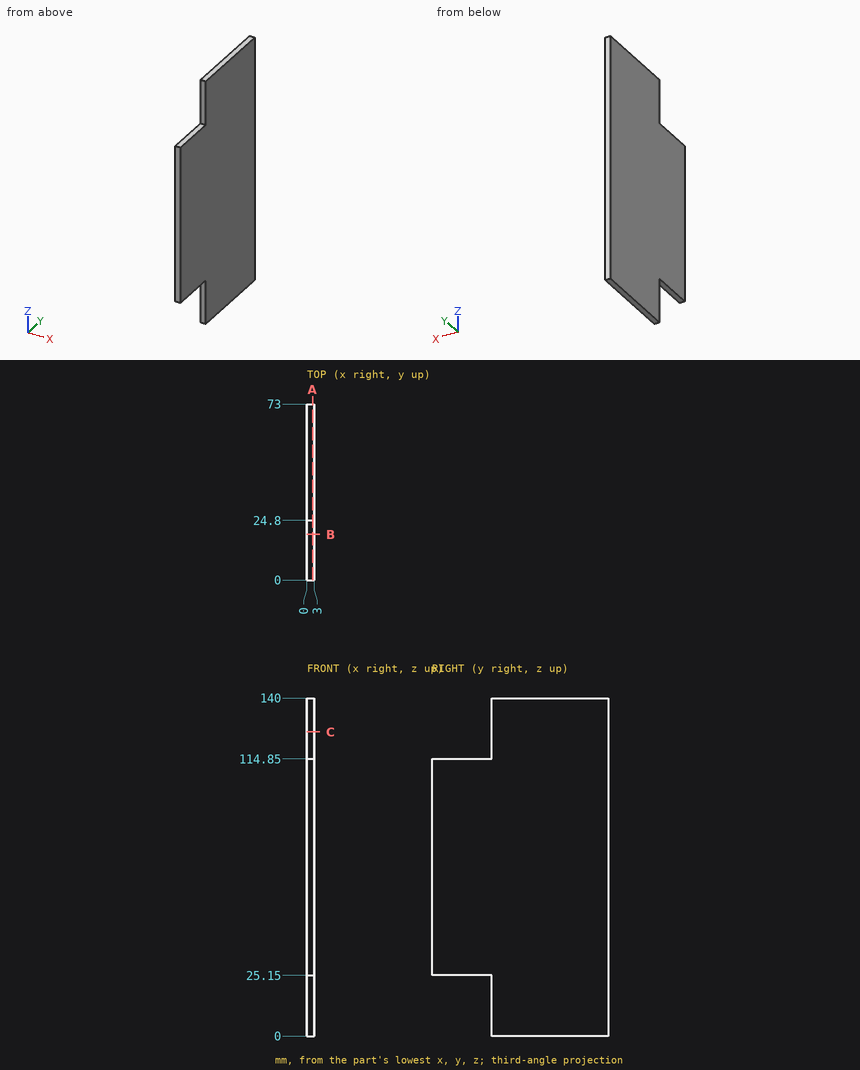
Can you work these out from the drawing? Everything is in mm from the part's minimum corner. Round coordinates to 2 decimals unless told otherwise and drop trailing zeros. Loops run counter-clockwise (first coordinate to the right, second up) from the corner with the lowest first, then second, coordinate; pieces in that order, holes last. Notation, with made-up numbers: (29, 76.5) - (78, 76.5) arc R18 ccw to (78, 96.5) - close; hole circle Ø5 at (73.5, 22). An arc over 180 degrees is marked (long way). Answer in a Markdown table with one row per item. Add a question column.
Q1. I want a section at B-B on y = 19. List the corners of the cut face in (x, z) for me, and give its area (3 significant figures).
Q2. I want a section at C-C on z = 126. List the corners of the cut face in (x, y) for me, and give its area (3 significant figures).
Q3. I need wall thicknesses on L1, parallel to Y at x = 2.3, z = 122.5; L2, parallel to Z at x = 1.25, y = 9. Which ranges of each line are inside material? Lowest first, please.
Q4. I want a section at A-A on x = 2.4. List the corners of the cut face in (y, z) for me, and give its area (3 significant figures).
Q5. For pin 1 Ø0.9 at (x, z) = (1.5, 6.5) entering from -Y; pin 2 Ø1.5 at (x, y) = (1, 15.5) entering from -Z, each with a flat end and sliding along its axis, tell me the tip position at first contact or that it passes through.
A:
| question | item | result |
|---|---|---|
| 1 | outline | (0, 25.15) - (3, 25.15) - (3, 114.85) - (0, 114.85) - close |
| 1 | area | 269 mm^2 |
| 2 | outline | (0, 24.8) - (3, 24.8) - (3, 73) - (0, 73) - close |
| 2 | area | 145 mm^2 |
| 3 | L1 | 24.8 to 73 |
| 3 | L2 | 25.15 to 114.85 |
| 4 | outline | (0, 25.15) - (24.8, 25.15) - (24.8, 0) - (73, 0) - (73, 140) - (24.8, 140) - (24.8, 114.85) - (0, 114.85) - close |
| 4 | area | 8,970 mm^2 |
| 5 | pin 1 | y = 24.8 |
| 5 | pin 2 | z = 25.15 |
